Here's how the part is built. I have some questions about the finished solid (model axes, mm). Face numbers are marked on the shaded views. A direction names the side the tool comes from. Give positions to 0.01 mm unless a question says otherwise; leave off trailing zeros. Write each loop counter-clockwise with the first axis right and the second up, starting at its lowest first coordinate (ties: lowest second). Pieces come first, ordered by that corner, then holes. Notation, with made-up numbers: (28.5, 51.25) -> (63.5, 51.25) arc R8 ccw to (63.5, 66.25) -> close; hole circle Ø6 at (21.25, 69). An arc over 180 degrees is marked (long way). Return JSON: item names as keys, results as strings.
from build123d import *
from build123d.topology import SkipClean

# Parameters (mm, degrees)
SWEEP_THIN1_PROFILE_R   = 14.605
SWEEP_THIN1_PROFILE_R_2 = 9.525
SKETCH15_R              = 12.065
SKETCH15_R_2            = 9.525
BOSS_EXTRUDE2_DEPTH     = 9.525


with BuildPart() as part:
    # Sweep-Thin1: sweep along a curve in space
    with BuildLine() as sweep_thin1_path:
        Line((-66.675, 0, 0), (66.675, 0, 0))
    # Sweep-Thin1 profile (on start of the path) → Sweep-Thin1 (sweep)
    with BuildSketch(Plane(origin=(-66.675, 0, 0), x_dir=(0, 0, 1), z_dir=(1, 0, 0))):
        Circle(SWEEP_THIN1_PROFILE_R)
        Circle(SWEEP_THIN1_PROFILE_R_2, mode=Mode.SUBTRACT)
    sweep(path=sweep_thin1_path.line)

    # Sketch15 → Boss-Extrude2 (add)
    with SkipClean():  # the faces are left unmerged after this step: merging them gives an invalid solid
        with BuildSketch(Plane.ZY.offset(66.675)):
            with Locations(Location((0, 0, 0), (0, 0, 180))):
                Circle(SKETCH15_R)
            with Locations(Location((0, 0, 0), (0, 0, 180))):
                Circle(SKETCH15_R_2, mode=Mode.SUBTRACT)
        boss_extrude2 = extrude(amount=BOSS_EXTRUDE2_DEPTH)
    add(part.part.scale(1), mode=Mode.REPLACE)  # the faces are merged on a copy

    # Mirror1: Boss-Extrude2 across plane
    with SkipClean():  # the faces are left unmerged after this step: merging them gives an invalid solid
        add(boss_extrude2.mirror(Plane(origin=(0, 0, 0), x_dir=(0, 0, 1), z_dir=(1, 0, 0))))


solid = part.part
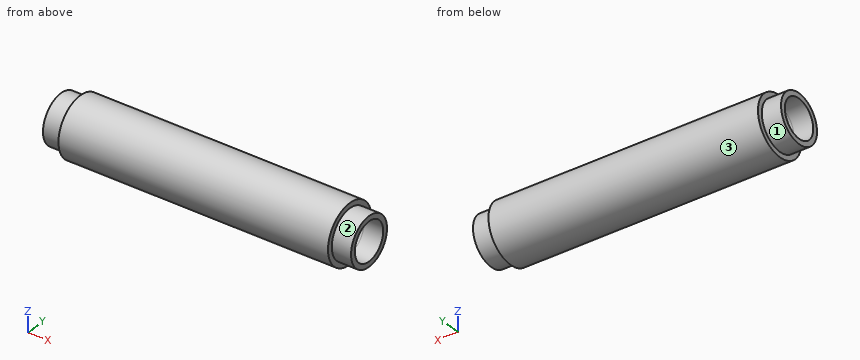
1. Suppose I cut it at C-C, the plane x = 64. List the corners of the cut face in (y, z) for me (3 decimals).
Taken from the geometry:
{"outline": "circle Ø29.21 at (0, 0); hole circle Ø19.05 at (0, 0)"}
2. If I drill on line 1 (Y direction, x = 69.5, z = 0) (3 decimals); line 2 (Y direction, x = 29, z = 0) (3 decimals); line 3 (Z direction, x = -58, y = 6.75), over which ranges is the centre line in solid material (lowest first)? Write a range as [from, to].
Taken from the geometry:
{"line 1": "y = [-12.065, -9.525], [9.525, 12.065]", "line 2": "y = [-14.605, -9.525], [9.525, 14.605]", "line 3": "z = [-12.95, -6.72], [6.72, 12.95]"}
3. Suppose I cut it at A-A, the plane z = 0. List the corners of the cut face in (x, y) for me (3 decimals).
Taken from the geometry:
{"outline": "(-76.2, -12.065) -> (-66.675, -12.065) -> (-66.675, -14.605) -> (66.675, -14.605) -> (66.675, -12.065) -> (76.2, -12.065) -> (76.2, -9.525) -> (-76.2, -9.525) -> close; (-76.2, 9.525) -> (76.2, 9.525) -> (76.2, 12.065) -> (66.675, 12.065) -> (66.675, 14.605) -> (-66.675, 14.605) -> (-66.675, 12.065) -> (-76.2, 12.065) -> close"}
4. For pin 1 Ø5 at (y, z) = (10, -10.5) entering from +X; pin 2 Ø2 at (x, z) = (9.5, 2) entering from +Y; pin 3 Ø17 at (y, z) = (0, 0) entering from +X; pin 4 Ø1 at (x, z) = (-42, 5) entering from +Y, each with a flat end and sliding along its axis, tell me the tip position at first contact or that it passes through.
Taken from the geometry:
{"pin 1": "stops at x = 76.2", "pin 2": "stops at y = 14.57", "pin 3": "passes through", "pin 4": "stops at y = 13.89"}
5. Which directions (+Z, -Z, +X, -X, +Y, -Y) give clear straight access to the entire face, cutting with the end or side of a thin tool? Please do the marked faces 1, 2 and 3.
Taken from the geometry:
{"face 1": "-X", "face 2": "+X", "face 3": "+X, -X"}
